The drawing under review shows one solid part. Ordinate dimensions are in mm from its lowest x, y, z. A direction names the side the tool comes from. Coordinates: 2 decimals unless noted, no trailing zeros. Write each loop counter-clockwise with the first axis right and the second up, starting at its lowest first coordinate (ties: lowest second). Pieces come first, ordered by that corner, then holes.
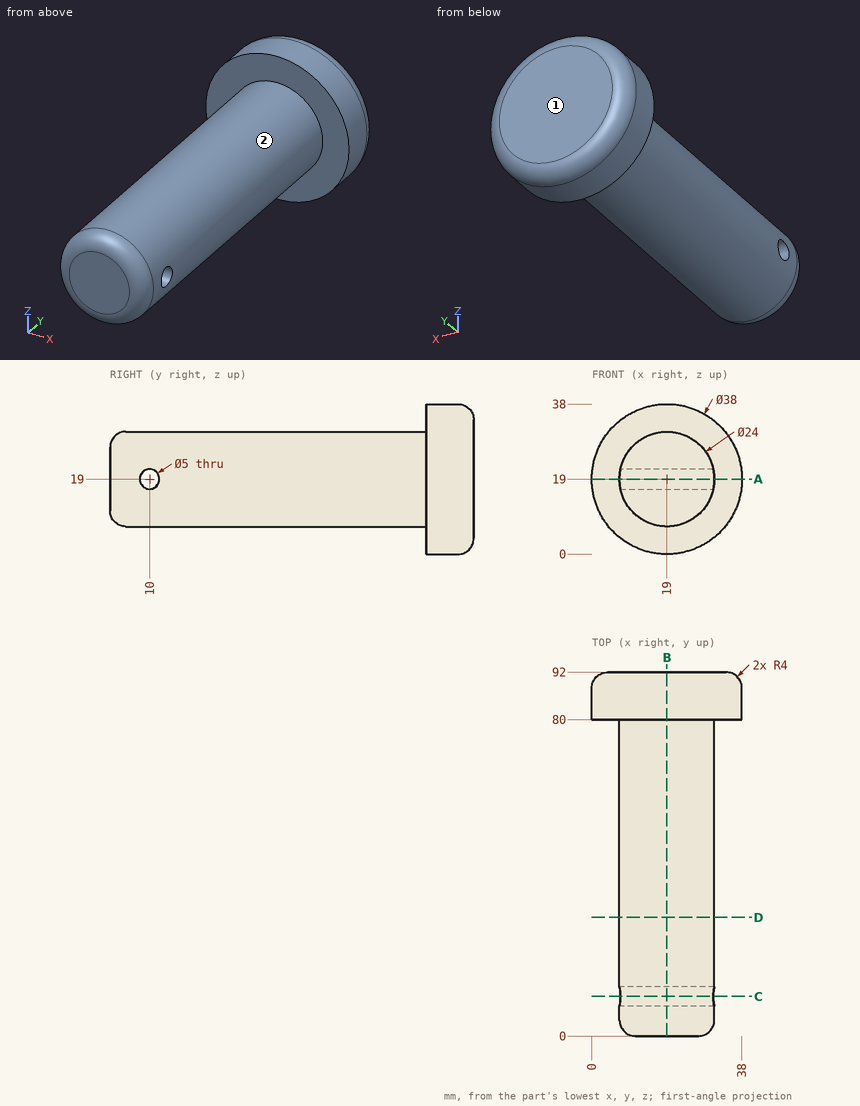
Q1. Clearance check with flat-ended pins moving along their axes: pin 1 Ø6 at (y, z) = (10, 19) entering from +X; pin 2 Ø8 at (y, z) = (71.5, 25) entering from +X; pin 3 Ø3 at (x, z) = (13.5, 8.5) entering from -Y; pin 4 Ø3 at (y, z) = (64.5, 4.5) entering from +X. State where each tip first meets the part, or that it passes through.
Ans:
pin 1: stops at x = 31
pin 2: stops at x = 30.83
pin 3: stops at y = 0.77
pin 4: passes through
Q2. Add section B-B (x = 19). State the section outline as (y, z) points.
Ans:
outline: (0, 11) arc R4 ccw to (4, 7) - (80, 7) - (80, 0) - (88, 0) arc R4 ccw to (92, 4) - (92, 34) arc R4 ccw to (88, 38) - (80, 38) - (80, 31) - (4, 31) arc R4 ccw to (0, 27) - close; hole circle Ø5 at (10, 19)
Q3. Add section A-A (z = 19). State the section outline as (x, y) points.
Ans:
outline: (0, 80) - (7, 80) - (7, 12.5) - (31, 12.5) - (31, 80) - (38, 80) - (38, 88) arc R4 ccw to (34, 92) - (4, 92) arc R4 ccw to (0, 88) - close; (7, 4) arc R4 ccw to (11, 0) - (27, 0) arc R4 ccw to (31, 4) - (31, 7.5) - (7, 7.5) - close
Q4. Add section D-D (y = 30). State the section outline as (x, z) points.
Ans:
outline: circle Ø24 at (19, 19)
Q5. Add section C-C (y = 10). State the section outline as (x, z) points.
Ans:
outline: (7.26, 16.5) arc R12 ccw to (30.74, 16.5) - close; (7.26, 21.5) - (30.74, 21.5) arc R12 ccw to start
Q6. Tool access review of the marked faces 1 and 2: name each direction out of +Z, -Z, +X, -X, +Y, -Y from which nothing blocks a thin tool from reaching the whole face with its end or side.
Ans:
face 1: +Z, -Z, +X, -X, +Y
face 2: -Y
Q7. For probe 1 along Y at (x, z) = (21, 19); probe 2 along Y at (x, z) = (9, 27); probe 3 along Z at (x, y) = (20.5, 12), list the stretches that pass through material, from the lowest coordinate up.
Ans:
probe 1: y = 0 to 7.5, 12.5 to 92
probe 2: y = 80 to 92
probe 3: z = 7.09 to 17.5, 20.5 to 30.91
